Geometry: final body of the model. Coordinates: model frame, mm. A direction names the side the tool comes from. Give positions to 0.01 mm unless a question says otherwise; leave off trailing zeros. Write each loop counter-clockwise with the first axis right and the second up, starting at its lowest first coordinate (ties: lowest second). Pieces come first, ordered by that corner, then holes. Notation, with made-up numbers: M 75.5,9 L 83.5,9 A24 ccw 83.5,45 Z; hole C 4,71 d6. An arc over 180 degrees is marked long. Use a Markdown table: item, result. Add a question column.
1) Section A-A on x = -5.75. Return the cut outline in (y, z) (1 decimal), then the cut area to 3 significant figures.
2) Set-up query: faces 1 (the flat face through (12.7, 0, -5)), 2 (the flat face through (-11.112, 0, -5)). Return all of +Z, -Z, +X, -X, +Y, -Y with unobstructed straight access to the full face (end or side cutting, diameter ignored); none if empty.
3) Pin query (flat end, axial travel): pin 1 (3 mm diameter, centred on x = 0, z = -374.65, fed in from -Y). Return the tip coordinate at first contact, or that it passes through.
4) Line query: line 1 (Z direction, x = 0, y = -12.1) (1 decimal); line 2 (Y direction, x = 8, z = -2); line 3 (X direction, y = 11.8, z = 355.6). Output: solid intervals per line, ascending.
5) Section B-B on z = -33. Return the cut outline in (x, y), then the cut area to 3 significant figures.
6) Draft query along X for faces 3 (the flat face through (0, 11.112, -5)), 4 (the flat face through (0, 12.7, -5)), 5 (the flat face through (11.112, 0, -5)), 6 (the flat face through (-12.7, 0, -5)). Return one class per face: +X half, -X half, draft (parallel to the pull), parting line (faces both ways), or undercut.
Autodesk Inventor part; units mm, degrees
ref_plane "YZ Plane" through (0, 0, 0) normal (1, 0, 0) x (0, 1, 0)
ref_plane "XZ Plane" through (0, 0, 0) normal (0, 1, 0) x (-1, 0, 0)
ref_plane "XY Plane" through (0, 0, 0) normal (0, 0, 1) x (1, 0, 0)
sketch "Sketch1" plane through (0, 0, 0) normal (0, 0, 1) x (1, 0, 0)
  line L0 (0, 0) -> (-11.1125, 0) construction
  line L1 (0, 0) -> (0, 11.1125) construction
  line L2 (-11.1125, 11.1125) -> (11.1125, 11.1125)
  line L3 (11.1125, 11.1125) -> (11.1125, -11.1125)
  line L4 (11.1125, -11.1125) -> (-11.1125, -11.1125)
  line L5 (-11.1125, -11.1125) -> (-11.1125, 11.1125)
  line L6 (-12.7, 12.7) -> (12.7, 12.7)
  line L7 (12.7, 12.7) -> (12.7, -12.7)
  line L8 (12.7, -12.7) -> (-12.7, -12.7)
  line L9 (-12.7, -12.7) -> (-12.7, 12.7)
  line L10 (-11.1125, 0) -> (-12.7, 0) construction
  line L11 (0, 11.1125) -> (0, 12.7) construction
  dimension "d0" = 25.4
  dimension "d1" = 1.5875
extrude "Extrusion1" add sketch "Sketch1" along normal mid plane 768.35
sketch "Sketch3" plane through (-12.7, -12.7, 384.175) normal (0, -1, 0) x (1, 0, 0)
  line L0 (12.7, -384.175) -> (0, -384.175) construction
  line L1 (0, -768.35) -> (0, 0) construction
  line L2 (12.7, -384.175) -> (12.7, 0) construction
  circle A0 centre (12.7, -9.525) radius 1.5875
  circle A1 centre (12.7, -28.575) radius 1.5875
  line L3 (0, 0) -> (25.4, 0)
  circle A2 centre (12.7, -758.825) radius 1.5875
  circle A3 centre (12.7, -739.775) radius 1.5875
  dimension "d9" = 3.175
  dimension "d10" = 9.525
  dimension "d11" = 19.05
extrude "Extrusion3" cut sketch "Sketch3" against normal through all
properties part number "Long Side" material "Aluminum 6061"
Found:
| question | item | result |
|---|---|---|
| 1 | outline | M -12.7,-384.2 L -11.1,-384.2 L -11.1,384.2 L -12.7,384.2 Z; M 11.1,-384.2 L 12.7,-384.2 L 12.7,384.2 L 11.1,384.2 Z |
| 1 | area | 2,440 mm² |
| 2 | face 1 | +Z, -Z, +X, +Y, -Y |
| 2 | face 2 | +Z, -Z |
| 3 | pin 1 | through |
| 4 | line 1 | -384.2 to -376.2, -373.1 to -357.2, -354 to 354, 357.2 to 373.1, 376.2 to 384.2 |
| 4 | line 2 | -12.7 to -11.11, 11.11 to 12.7 |
| 4 | line 3 | -12.7 to -1.59, 1.59 to 12.7 |
| 5 | outline | M -12.7,-12.7 L 12.7,-12.7 L 12.7,12.7 L -12.7,12.7 Z; hole M -11.11,-11.11 L 11.11,-11.11 L 11.11,11.11 L -11.11,11.11 Z |
| 5 | area | 151 mm² |
| 6 | face 3 | undercut |
| 6 | face 4 | draft |
| 6 | face 5 | undercut |
| 6 | face 6 | -X half |
